Geometry: final body of the model. Coordinates: model frame, mm. A direction names the side the tool comes from. Round coordinates to 2 decimals unless told otherwise and drop trailing zeros. Loops run counter-clockwise (first coordinate to the right, second up) from the corner with the lowest first, then second, coordinate; pieces in that order, holes last. Notation, with made-up numbers: M -38,64.25 L -27,64.25 A13 cw -27,68.25 Z; hole C -29,-36.5 d2. An arc over 180 degrees is marked long. Return JSON: item names as keys, results as strings.
from build123d import *

# Parameters (mm, degrees)
F0_R     = 28.575
F0_R_2   = 25.4
F1_DEPTH = 25.4
F2_R     = 63.5
F3_DEPTH = 6.35
F4_R     = 2.54
F5_R     = 4.92125
F6_DEPTH = 6.35


with BuildPart() as f1:
    # F0 (on Top) → F1 (new body)
    with BuildSketch(Plane.XY):
        Circle(F0_R)
        Circle(F0_R_2, mode=Mode.SUBTRACT)
    extrude(amount=F1_DEPTH)

    # F2 (on Top) → F3 (join)
    with BuildSketch(Plane.XY):
        Circle(F2_R)
    extrude(amount=-F3_DEPTH)

    # F4
    f4_edges = [f1.edges().sort_by_distance(p)[0] for p in [
        (-63.5, 0, 0),
        (-28.575, 0, 0),
    ]]
    fillet(f4_edges, radius=F4_R)

    # F5 (on face) → F6 (cut, through all)
    with BuildSketch(Plane.XY):
        with Locations((50.8, 0)):
            Circle(F5_R)
        with Locations((0, -50.8)):
            Circle(F5_R)
        with Locations((-50.8, 0)):
            Circle(F5_R)
        with Locations((0, 50.8)):
            Circle(F5_R)
    extrude(amount=-F6_DEPTH, mode=Mode.SUBTRACT)


solid = f1.part
Q1. Section query C-C (z = 16.5). Output: boundary loops of the cut face in (x, y) (3 decimals).
Determined:
{"outline": "C 0,0 d57.15; hole C 0,0 d50.8"}
Q2. Material intervals for L1, parallel to Y at x = 0, z = -4; L2, parallel to X at y = -0.5, z = 24.5; L3, parallel to Z at x = -37, y = 28, sorted ascending.
Determined:
{"L1": "y = -63.5 to -55.72, -45.88 to 45.88, 55.72 to 63.5", "L2": "x = -28.57 to -25.4, 25.4 to 28.57", "L3": "z = -6.35 to 0"}
Q3. Section query A-A (x = 0). Output: boundary loops of the cut face in (y, z) (3 decimals).
Determined:
{"outline": "M -63.5,-6.35 L -55.721,-6.35 L -55.721,0 L -60.96,0 A2.54 ccw -63.5,-2.54 Z; M -45.879,-6.35 L 45.879,-6.35 L 45.879,0 L 31.115,0 A2.54 cw 28.575,2.54 L 28.575,25.4 L 25.4,25.4 L 25.4,0 L -25.4,0 L -25.4,25.4 L -28.575,25.4 L -28.575,2.54 A2.54 cw -31.115,0 L -45.879,0 Z; M 55.721,-6.35 L 63.5,-6.35 L 63.5,-2.54 A2.54 ccw 60.96,0 L 55.721,0 Z"}
Q4. Pin query (flat end, axial travel): pin 1 (1 mm diameter, centred on x = 18, z = 18.5, fed in from -Y); pin 2 (12 mm diameter, centred on x = 16, z = 16, fed in from -Y); pin 3 (1 mm diameter, centred on x = 29.5, z = 1.5, fed in from +Y); pin 4 (4 mm diameter, centred on x = 29, y = 17.5, fed in from +Z). Return the tip coordinate at first contact, or that it passes through.
Determined:
{"pin 1": "stops at y = -22.59", "pin 2": "stops at y = -26.77", "pin 3": "passes through", "pin 4": "stops at z = 0"}
Q5. Pull-direction query (X, two-part tool) for faces 3 (the cylindrical face through (2.271, 46.434, -3.131)), 4 (the cylindrical face through (-28.547, 1.256, 13.81)), 5 (the flat face through (-28, 14, 0)); classes: pulls with the +X half, pulls with the -X half, needs draft (parallel to the pull), parting line crosses it, or undercut.
Determined:
{"face 3": "undercut", "face 4": "parting line crosses it", "face 5": "needs draft"}
Q6. Reachability of faces 1 (the flat face through (0, 0, 0)), 2 (the flat face through (-26, -2, 25.4)) from +Z, -Z, +X, -X, +Y, -Y: full face, straight path, thin tool, end or side. Return the list, or none.
Determined:
{"face 1": "+Z", "face 2": "+Z, +X, -X, +Y, -Y"}
